from build123d import *

# Parameters (mm, degrees)
SKETCH1_W                        = 95
SKETCH1_H                        = 95
BOSS_EXTRUDE1_DEPTH              = 60
SKETCH2_W                        = 95
SKETCH2_H                        = 5
BOSS_EXTRUDE2_DEPTH              = 25.4
FILLET1_R                        = 5
F_1_4_CLEARANCE_HOLE1_AT_2_COUNT = 2
F_1_4_CLEARANCE_HOLE1_AT_2_PITCH = 69.6
BOSS_EXTRUDE3_DEPTH              = 3
CHAMFER1_SIZE                    = 5
CHAMFER1_SIZE_2                  = 3.004303095
SKETCH6_W                        = 50
SKETCH6_H                        = 44
CUT_EXTRUDE1_DEPTH               = 51
SKETCH6_3_R                      = 12.5
CUT_EXTRUDE2_DEPTH               = 106.69134307
SKETCH7_W                        = 5
SKETCH7_H                        = 44
BOSS_EXTRUDE4_DEPTH              = 27
SKETCH8_W                        = 5
SKETCH8_H                        = 12.5
BOSS_EXTRUDE5_DEPTH              = 24
CBORE_FOR_M3_SBHCS1_D            = 3.4
CBORE_FOR_M3_SBHCS1_CBORE_D      = 6.7
CBORE_FOR_M3_SBHCS1_CBORE_DEPTH  = 1.65
CHAMFER2_SIZE                    = 5
CHAMFER3_SIZE                    = 5
F_6_0MM_DOWEL_HOLE1_D            = 5.5
F_6_0MM_DOWEL_HOLE1_DEPTH        = 12
F_6_0MM_DOWEL_HOLE1_TIP          = 1.652366702
F_3_0MM_DOWEL_HOLE1_D            = 3.5
F_3_0MM_DOWEL_HOLE1_DEPTH        = 12
F_3_0MM_DOWEL_HOLE1_TIP          = 1.051506083


with BuildPart() as part:
    # Sketch1 → Boss-Extrude1 (new body)
    with BuildSketch(Plane(origin=(0, 0, 0), x_dir=(1, 0, 0), z_dir=(0, 1, 0))):
        Rectangle(SKETCH1_W, SKETCH1_H)
    extrude(amount=BOSS_EXTRUDE1_DEPTH)

    # Sketch2 → Boss-Extrude2 (add)
    with BuildSketch(Plane.XY.offset(47.5)):
        with Locations((0, 2.5)):
            Rectangle(SKETCH2_W, SKETCH2_H)
    boss_extrude2 = extrude(amount=BOSS_EXTRUDE2_DEPTH)

    # Mirror1: Boss-Extrude2 across plane
    add(boss_extrude2.mirror(Plane.XY))

    # Fillet1
    fillet1_edges = [part.edges().sort_by_distance(p)[0] for p in [
        (-47.5, 2.5, 72.9),
        (47.5, 2.5, 72.9),
        (-47.5, 2.5, -72.9),
        (47.5, 2.5, -72.9),
        (47.5, 32.5, 47.5),
        (-47.5, 32.5, 47.5),
        (-47.5, 32.5, -47.5),
        (47.5, 32.5, -47.5),
    ]]
    fillet(fillet1_edges, radius=FILLET1_R)

    # Sketch4 → 1/4 Clearance Hole1 (revolve, cut)
    with BuildSketch(Plane(origin=(34.8, 5, 60.2), x_dir=(0, 0, 1), z_dir=(1, 0, 0))):
        Polygon((0, 0), (0, 12.029827343), (3.3782, 10), (3.3782, 0), align=None)
    f_1_4_clearance_hole1 = revolve(axis=Axis((34.8, 11.35, 60.2), (0, -1, 0)), mode=Mode.SUBTRACT)

    # 1/4 Clearance Hole1 at 2: 1/4 Clearance Hole1 ×2
    with Locations(*[(-i * F_1_4_CLEARANCE_HOLE1_AT_2_PITCH, 0, 0) for i in range(1, F_1_4_CLEARANCE_HOLE1_AT_2_COUNT)]):
        add(f_1_4_clearance_hole1, mode=Mode.SUBTRACT)

    # Mirror2: 1/4 Clearance Hole1 across plane
    add(f_1_4_clearance_hole1.mirror(Plane.XY), mode=Mode.SUBTRACT)

    # Mirror2 copy 1 sketch → Mirror2 copy 1 (revolve, cut)
    with BuildSketch(Plane(origin=(-34.8, 5, -60.2), x_dir=(0, 0, -1), z_dir=(1, 0, 0))):
        Polygon((0, 0), (0, -12.029827343), (3.3782, -10), (3.3782, 0), align=None)
    revolve(axis=Axis((-34.8, 11.35, -60.2), (0, 1, 0)), mode=Mode.SUBTRACT)

    # Sketch5 → Boss-Extrude3 (add)
    with BuildSketch(Plane(origin=(0, 0, -47.5), x_dir=(-1, 0, 0), z_dir=(0, 0, -1))):
        Polygon((0, 60), (-2.886751346, 55), (2.886751346, 55), align=None)
    extrude(amount=BOSS_EXTRUDE3_DEPTH)

    # Chamfer1
    # the kernel refuses this chamfer: 5, 3.004303095 mm, written as the material it adds along each edge
    with BuildSketch(Plane(origin=(15.817899449, 55, -47.5), x_dir=(0, -0.9998016840798124, 0.01991463058083395), z_dir=(-1, 0, 0))) as chamfer1_piece_1_section:
        Polygon((CHAMFER1_SIZE * 0.99980168408, -CHAMFER1_SIZE * 0.0199146305808), (-CHAMFER1_SIZE_2 * 0.0199146305817, -CHAMFER1_SIZE_2 * 0.999801684126), (0, 0), align=None)
    chamfer1_piece_1 = extrude(amount=31.635798898, mode=Mode.PRIVATE)
    chamfer1_piece_1 = split(chamfer1_piece_1, bisect_by=Plane(origin=(-2.998221353, 54.806928285, -48.382310959), z_dir=(0.8660254037844363, -0.5000000000000041, 0)), keep=Keep.TOP, mode=Mode.PRIVATE)
    chamfer1_piece_1 = split(chamfer1_piece_1, bisect_by=Plane(origin=(2.998221353, 54.806928285, -48.382310959), z_dir=(-0.8660254037844365, -0.5000000000000039, 0)), keep=Keep.TOP, mode=Mode.PRIVATE)
    chamfer1_piece_1 = split(chamfer1_piece_1, bisect_by=Plane(origin=(0, 53.07590438, -50.5), z_dir=(0, 0, 1)), keep=Keep.TOP, mode=Mode.PRIVATE)
    add(chamfer1_piece_1)

    # Sketch6 → Cut-Extrude1 (cut)
    with BuildSketch(Plane.XZ):
        with Locations((-22.5, 0)):
            Rectangle(SKETCH6_W, SKETCH6_H)
    extrude(amount=-CUT_EXTRUDE1_DEPTH, mode=Mode.SUBTRACT)

    # Sketch6<3> → Cut-Extrude2 (cut, through all)
    with BuildSketch(Plane.XZ):
        with Locations(Location((-19.5, 0, 0), (0, 0, 270))):
            Circle(SKETCH6_3_R)
    extrude(amount=-CUT_EXTRUDE2_DEPTH, mode=Mode.SUBTRACT)

    # Sketch7 → Boss-Extrude4 (add)
    with BuildSketch(Plane.XZ.offset(-51)):
        with Locations((-45, 0)):
            Rectangle(SKETCH7_W, SKETCH7_H)
    extrude(amount=BOSS_EXTRUDE4_DEPTH)

    # Sketch8 → Boss-Extrude5 (add)
    with BuildSketch(Plane.XZ.offset(-24)):
        with Locations((-45, -15.75)):
            Rectangle(SKETCH8_W, SKETCH8_H)
        with Locations((-45, 15.75)):
            Rectangle(SKETCH8_W, SKETCH8_H)
    extrude(amount=BOSS_EXTRUDE5_DEPTH)

    # CBORE for M3 SBHCS1 (through all)
    with Locations(Plane(origin=(0, 60, 0), x_dir=(1, 0, 0), z_dir=(0, 1, 0))):
        with Locations((-19.5, 0), (-4, -15.5), (-35, 15.5), (-35, -15.5), (-4, 15.5)):
            CounterBoreHole(CBORE_FOR_M3_SBHCS1_D / 2, CBORE_FOR_M3_SBHCS1_CBORE_D / 2, CBORE_FOR_M3_SBHCS1_CBORE_DEPTH)

    # Chamfer2
    # the kernel refuses this chamfer: 5 mm, written as the material it adds along each edge
    with BuildSketch(Plane(origin=(42.5, 5, -47.5), x_dir=(0, 0.9996219169112969, 0.0274958766105808), z_dir=(-1, 0, 0))) as chamfer2_piece_1:
        Polygon((CHAMFER2_SIZE * 0.999621916911, CHAMFER2_SIZE * 0.0274958766106), (-CHAMFER2_SIZE * 0.0274958766106, CHAMFER2_SIZE * 0.999621916911), (0, 0), align=None)
    extrude(amount=85)
    with BuildSketch(Plane(origin=(42.5, 5, 47.5), x_dir=(0, 0.9996219169112968, -0.027495876610586324), z_dir=(-1, 0, 0))) as chamfer2_piece_2:
        Polygon((CHAMFER2_SIZE * 0.999621916911, -CHAMFER2_SIZE * 0.0274958766106), (-CHAMFER2_SIZE * 0.0274958766106, -CHAMFER2_SIZE * 0.999621916911), (0, 0), align=None)
    extrude(amount=85)
    with BuildSketch(Plane(origin=(-42.5, 5, 42.5), x_dir=(0, 0, 1), z_dir=(1, 0, 0))) as chamfer2_piece_3_section:
        Polygon((5, -CHAMFER2_SIZE), (5 + CHAMFER2_SIZE, 0), (5, 0), align=None)
    chamfer2_piece_3 = revolve(axis=Axis((-42.5, 5, 42.5), (0, -1, 0)), revolution_arc=237.405771779, mode=Mode.PRIVATE)
    chamfer2_piece_3 = split(chamfer2_piece_3, bisect_by=Plane(origin=(-47.5, 7.211903133, 46.338242127), z_dir=(1, 0, 0)), keep=Keep.TOP, mode=Mode.PRIVATE)
    add(chamfer2_piece_3)
    with BuildSketch(Plane(origin=(42.5, 5, 42.5), x_dir=(0, 0, 1), z_dir=(-1, 0, 0))) as chamfer2_piece_4_section:
        Polygon((5, CHAMFER2_SIZE), (5 + CHAMFER2_SIZE, 0), (5, 0), align=None)
    chamfer2_piece_4 = revolve(axis=Axis((42.5, 5, 42.5), (0, 1, 0)), revolution_arc=237.405771779, mode=Mode.PRIVATE)
    chamfer2_piece_4 = split(chamfer2_piece_4, bisect_by=Plane(origin=(47.5, 7.211903133, 46.338242127), z_dir=(-1, 0, 0)), keep=Keep.TOP, mode=Mode.PRIVATE)
    add(chamfer2_piece_4)
    with BuildSketch(Plane(origin=(42.5, 5, -42.5), x_dir=(0, 0, -1), z_dir=(-1, 0, 0))) as chamfer2_piece_5_section:
        Polygon((5 + CHAMFER2_SIZE, 0), (5, -CHAMFER2_SIZE), (5, 0), align=None)
    chamfer2_piece_5 = revolve(axis=Axis((42.5, 5, -42.5), (0, -1, 0)), revolution_arc=237.405771779, mode=Mode.PRIVATE)
    chamfer2_piece_5 = split(chamfer2_piece_5, bisect_by=Plane(origin=(47.5, 6.474161158, -49.057149182), z_dir=(-1, 0, 0)), keep=Keep.TOP, mode=Mode.PRIVATE)
    add(chamfer2_piece_5)
    with BuildSketch(Plane(origin=(-42.5, 5, -42.5), x_dir=(0.8425066666450718, 0, 0.5386859165215014), z_dir=(0.5386859165215014, 0, -0.8425066666450718))) as chamfer2_piece_6_section:
        Polygon((5 + CHAMFER2_SIZE, 0), (5, -CHAMFER2_SIZE), (5, 0), align=None)
    chamfer2_piece_6 = revolve(axis=Axis((-42.5, 5, -42.5), (0, -1, 0)), revolution_arc=237.405771779, mode=Mode.PRIVATE)
    chamfer2_piece_6 = split(chamfer2_piece_6, bisect_by=Plane(origin=(-47.5, 7.211903133, -46.338242127), z_dir=(1, 0, 0)), keep=Keep.TOP, mode=Mode.PRIVATE)
    add(chamfer2_piece_6)

    # Chamfer3
    chamfer3_edges = [part.edges().sort_by_distance(p)[0] for p in [
        (-45, 0, -9.5),
        (-45, 0, 9.5),
    ]]
    chamfer(chamfer3_edges, length=CHAMFER3_SIZE)

    # Ø6.0mm Dowel Hole1
    with Locations(Plane(origin=(0, 60, 0), x_dir=(1, 0, 0), z_dir=(0, 1, 0))):
        with Locations((0, 0), (39.952317218, 41.093696451), (-39.952317218, -41.093696451), (-39.952317218, 41.093696451), (39.952317218, -41.093696451)):
            Hole(F_6_0MM_DOWEL_HOLE1_D / 2, depth=F_6_0MM_DOWEL_HOLE1_DEPTH)
            with Locations((0, 0, -(F_6_0MM_DOWEL_HOLE1_DEPTH + F_6_0MM_DOWEL_HOLE1_TIP / 2))):  # 118° drill point
                Cone(0, F_6_0MM_DOWEL_HOLE1_D / 2, F_6_0MM_DOWEL_HOLE1_TIP, mode=Mode.SUBTRACT)

    # Ø3.0mm Dowel Hole1
    with Locations(Plane.XY.offset(47.5)):
        with Locations((-3.5, 50.7), (-12.8, 50.7)):
            Hole(F_3_0MM_DOWEL_HOLE1_D / 2, depth=F_3_0MM_DOWEL_HOLE1_DEPTH)
            with Locations((0, 0, -(F_3_0MM_DOWEL_HOLE1_DEPTH + F_3_0MM_DOWEL_HOLE1_TIP / 2))):  # 118° drill point
                Cone(0, F_3_0MM_DOWEL_HOLE1_D / 2, F_3_0MM_DOWEL_HOLE1_TIP, mode=Mode.SUBTRACT)


solid = part.part
Can you work these out from the model? Positions are in its coordinate system, mm. A direction names the side the tool comes from. Round coordinates to 2 decimals unless told otherwise and drop trailing zeros. Loops run counter-clockwise (first coordinate to the right, second up) from the corner with the lowest first, then second, coordinate; pieces in that order, holes last. Notation, with made-up numbers: (59, 24.5) - (82, 24.5) arc R34 ccw to (82, 59.5) - close; hole circle Ø10 at (45.5, -19.75). An arc over 180 degrees is marked (long way). Answer in a Markdown table with one row per item. Add a question column.
Q1. For pin 1 Ø3 at (x, y) = (-3.5, 50.7) entering from -Z; pin 2 Ø1 at (x, y) = (-4.5, 40.5) entering from +Z; pin 3 Ø3.5 at (x, z) = (-34, 16.5) entering from +Y; pin 4 Ø22.5 at (x, z) = (-19.5, 0) entering from -Y, each with a flat end and sliding along its axis, tell me the tip position at first contact or that it passes through.
Q2. I want a section at B-B on z = 60.2. List the corners of the cut face in (x, y) for me, and give its area (3 significant figures).
Q3. I need wall thicknesses on L1, parallel to X at y = 37, z = -20; L2, parallel to Z at x = -9, y = 13.5; L3, parallel to X at y = 59.3, z = 15.5. Which ranges of each line are inside material? Lowest first, please.
Q4. I want a section at D-D on y = 27. List the corners of the cut face in (x, z) for me.
Q5. We'd pull the mould along X, two halves only. Please class faces 5 (the cylindrical face through (-33.199, 59.187, -18.325)), 6 (the flat face through (47.5, 30, 1)), 7 (the flat face through (0.081, 51.907, -48.646)): pulls with the +X half, pulls with the -X half, needs draft (parallel to the pull), parting line crosses it, or undercut.
Q6. I want a section at C-C on x = -19.5. List the corners of the cut face in (y, z) for me, and give its area (3 significant figures).
Q7. I want a section at A-A on x = 34.8. List the corners of the cut face in (y, z) for me.
Q8. Which directions (+Z, -Z, +X, -X, +Y, -Y) give clear straight access to the entire face, cutting with the end or side of a thin tool? Please do faces 1 (the flat face through (0, 57, -50.5)), 2 (the flat face through (-1, 35, 47.5)), 3 (the flat face through (-20, 25, -22)), 4 (the flat face through (-45, 2.5, 12)).
A:
| question | item | result |
|---|---|---|
| 1 | pin 1 | z = -48.82 |
| 1 | pin 2 | z = 47.5 |
| 1 | pin 3 | y = 58.35 |
| 1 | pin 4 | through |
| 2 | outline | (-47.5, 0) - (-38.18, 0) - (-38.18, 5) - (-47.5, 5) - close; (-31.42, 0) - (31.42, 0) - (31.42, 5) - (-31.42, 5) - close; (38.18, 0) - (47.5, 0) - (47.5, 5) - (38.18, 5) - close |
| 2 | area | 407 mm^2 |
| 3 | L1 | -47.5 to -42.5, 2.5 to 47.5 |
| 3 | L2 | -47.5 to -22, 22 to 47.5 |
| 3 | L3 | -47.5 to -38.35, -31.65 to -7.35, -0.65 to 47.5 |
| 4 | outline | (-47.5, -42.5) arc R5 ccw to (-42.5, -47.5) - (42.5, -47.5) arc R5 ccw to (47.5, -42.5) - (47.5, 42.5) arc R5 ccw to (42.5, 47.5) - (-42.5, 47.5) arc R5 ccw to (-47.5, 42.5) - close; hole (-42.5, -22) - (2.5, -22) - (2.5, 22) - (-42.5, 22) - close |
| 5 | face 5 | undercut |
| 5 | face 6 | pulls with the +X half |
| 5 | face 7 | needs draft |
| 6 | outline | (0, -72.9) - (5, -72.9) - (5, -52.5) - (10, -47.5) - (60, -47.5) - (60, -12.5) - (51, -12.5) - (51, -22) - (0, -22) - close; (0, 22) - (51, 22) - (51, 12.5) - (60, 12.5) - (60, 47.5) - (10, 47.5) - (5, 52.5) - (5, 72.9) - (0, 72.9) - close |
| 6 | area | 3,510 mm^2 |
| 7 | outline | (0, -72.9) - (5, -72.9) - (5, -63.58) - (0, -63.58) - close; (0, -56.82) - (5, -56.82) - (5, -52.5) - (10, -47.5) - (60, -47.5) - (60, 47.5) - (10, 47.5) - (5, 52.5) - (5, 56.82) - (0, 56.82) - close; (0, 63.58) - (5, 63.58) - (5, 72.9) - (0, 72.9) - close |
| 8 | face 1 | -Z, +X, -X, +Y |
| 8 | face 2 | +Z, +X, -X, +Y |
| 8 | face 3 | -Y |
| 8 | face 4 | -X, -Y |
